Work out the finished part from the listing and answer in its coordinate system (mm). A direction names the side the tool comes from. Give positions to 0.01 mm unless a question says otherwise; leave off trailing zeros. Loops run counter-clockwise (first coordinate to the right, second up) from the corner with the lowest first, then second, coordinate; pieces in that order, holes last. Notation, with made-up numbers: (-16.5, -34.75) -> (-1.5, -34.75) arc R23 ccw to (-1.5, -4.75) -> close; hole circle Ø2 at (75.25, 24.25). An arc over 180 degrees is marked (long way). Answer as CSV lines item,"result". Start each with the question number.
1. Find section A-A, the plane z = 1.25. Give the vertices of the cut face in (x, y).
2. A tool of negligible diameter and unlimited length cuts with its end or side. For faces 1 (the face through (-20, 0, 2)), 2 (the face through (35, 0, 5)), 3 (the face through (-1, 5, 9)), 4 (the face through (-35, 0, 5)), from which of +Z, -Z, +X, -X, +Y, -Y can it reach the whole face along a straight path? Write none if from no direction.
3. Determine the mould class of faces 5 (the face through (-34.25, 0.08, 2.46)), 6 (the face through (28.4, 0.07, 5.86)), 7 (the face through (-28.4, 0.07, 5.86)), 8 (the face through (0, 0, 8)) for opening direction X: +X half, -X half, draft (parallel to the pull), parting line (faces both ways), or undercut.
4. Find section C-C, the plane x = 32.5. Give the vertices of the cut face in (y, z).
5. Flat-ended cylindrical pins translate along their axes: pin 1 Ø5 at (x, y) = (22, -1.5) entering from +Z; pin 2 Ø5 at (x, y) = (-33, -1) entering from +Z; pin 3 Ø4 at (y, z) = (-0.5, 9) entering from +X; pin 4 Ø5 at (x, y) = (-8, -1.5) entering from -Z. Find the tip coordinate at first contact, or state that the pin passes through.
6. Find the intervals of material crossed by line 1 along X through (y, z) = (-2, 2.75); line 2 along X through (y, z) = (-1.5, 3.75); line 3 along X through (y, z) = (-1.25, 4.25), in increasing order.
7. Find section D-D, the plane x = 19. Give the vertices of the cut face in (y, z), and give its area (3 significant figures).
8. Find section B-B, the plane y = 0. Give the vertices of the cut face in (x, z).
from build123d import *

# Parameters (mm, degrees)
SKETCH_W        = 75
SKETCH_H        = 10
PAD_DEPTH       = 15
SKETCH001_W     = 10
SKETCH001_H     = 10
POCKET_DEPTH    = 25
SKETCH002_R     = 1.75
POCKET001_DEPTH = 5
SKETCH003_W     = 40
SKETCH003_H     = 10
POCKET002_DEPTH = 8
FILLET_R        = 3
FILLET001_R     = 6
FILLET002_R     = 3
FILLET003_R     = 1


with BuildPart() as part:
    # Sketch → Pad (new body)
    with BuildSketch(Plane.XY):
        Rectangle(SKETCH_W, SKETCH_H)
    extrude(amount=PAD_DEPTH)

    # Sketch001 → Pocket (cut)
    with BuildSketch(Plane.XY.offset(5)):
        with Locations((-32.5, 0)):
            Rectangle(SKETCH001_W, SKETCH001_H)
        with Locations((32.5, 0)):
            Rectangle(SKETCH001_W, SKETCH001_H)
    extrude(amount=POCKET_DEPTH, mode=Mode.SUBTRACT)

    # Sketch002 → Pocket001 (cut)
    with BuildSketch(Plane.XY):
        with Locations((-32.5, 0)):
            Circle(SKETCH002_R)
        with Locations((32.5, 0)):
            Circle(SKETCH002_R)
    extrude(amount=POCKET001_DEPTH, mode=Mode.SUBTRACT)

    # Sketch003 → Pocket002 (cut)
    with BuildSketch(Plane.XY):
        Rectangle(SKETCH003_W, SKETCH003_H)
    extrude(amount=POCKET002_DEPTH, mode=Mode.SUBTRACT)

    # Fillet
    fillet_edges = [part.edges().sort_by_distance(p)[0] for p in [
        (-27.5, 0, 5),
        (27.5, 0, 5),
    ]]
    fillet(fillet_edges, radius=FILLET_R)

    # Fillet001
    fillet001_edges = [part.edges().sort_by_distance(p)[0] for p in [
        (-27.5, 0, 15),
        (27.5, 0, 15),
    ]]
    fillet(fillet001_edges, radius=FILLET001_R)

    # Fillet002
    fillet002_edges = [part.edges().sort_by_distance(p)[0] for p in [
        (-20, 0, 8),
        (20, 0, 8),
    ]]
    fillet(fillet002_edges, radius=FILLET002_R)

    # Fillet003
    fillet003_edges = [part.edges().sort_by_distance(p)[0] for p in [
        (-37.5, 0, 5),
        (-37.5, -5, 2.5),
        (-37.5, 5, 2.5),
        (37.5, -5, 2.5),
        (37.5, 0, 5),
        (37.5, 5, 2.5),
    ]]
    fillet(fillet003_edges, radius=FILLET003_R)


solid = part.part
Resolved:
1,outline,"(-37.5, -4) arc R1 ccw to (-36.5, -5) -> (-20, -5) -> (-20, 5) -> (-36.5, 5) arc R1 ccw to (-37.5, 4) -> close; (20, -5) -> (36.5, -5) arc R1 ccw to (37.5, -4) -> (37.5, 4) arc R1 ccw to (36.5, 5) -> (20, 5) -> close; hole circle Ø3.5 at (-32.5, 0); hole circle Ø3.5 at (32.5, 0)"
2,face 1,"-Z, +Y, -Y"
2,face 2,"+Z, +X, +Y, -Y"
2,face 3,"+Z, -Z, +X, -X, +Y"
2,face 4,"+Z, -X, +Y, -Y"
3,face 5,"undercut"
3,face 6,"+X half"
3,face 7,"-X half"
3,face 8,"undercut"
4,outline,"(-5, 0) -> (-1.75, 0) -> (-1.75, 5) -> (-5, 5) -> close; (1.75, 0) -> (5, 0) -> (5, 5) -> (1.75, 5) -> close"
5,pin 1,"stops at z = 15"
5,pin 2,"stops at z = 5"
5,pin 3,"stops at x = 27.67"
5,pin 4,"stops at z = 8"
6,line 1,"x = -37.5 to -20, 20 to 37.5"
6,line 2,"x = -37.5 to -33.4, -31.6 to -20, 20 to 31.6, 33.4 to 37.5"
6,line 3,"x = -37.47 to -33.72, -31.28 to -20, 20 to 31.28, 33.72 to 37.47"
7,outline,"(-5, 7.24) -> (5, 7.24) -> (5, 15) -> (-5, 15) -> close"
7,area,"77.6 mm^2"
8,outline,"(-37.5, 0) -> (-34.25, 0) -> (-34.25, 5) -> (-36.5, 5) arc R1 ccw to (-37.5, 4) -> close; (-30.75, 0) -> (-20, 0) -> (-20, 5) arc R3 cw to (-17, 8) -> (17, 8) arc R3 cw to (20, 5) -> (20, 0) -> (30.75, 0) -> (30.75, 5) -> (30.5, 5) arc R3 cw to (27.5, 8) -> (27.5, 9) arc R6 ccw to (21.5, 15) -> (-21.5, 15) arc R6 ccw to (-27.5, 9) -> (-27.5, 8) arc R3 cw to (-30.5, 5) -> (-30.75, 5) -> close; (34.25, 0) -> (37.5, 0) -> (37.5, 4) arc R1 ccw to (36.5, 5) -> (34.25, 5) -> close"
